The listing builds one solid part. Answer for the finished solid, in the listing's coordinates (mm). A direction names the side the tool comes from. Coordinates: 2 decimals unless noted, no trailing zeros. Order: outer loops, then holes, each group sorted by start corner. A loop starts at its lowest first (then second) coordinate and runs counter-clockwise, first axis right, second up. Notation, with made-up numbers: (1.25, -31) -> (28.25, -31) arc R33 cw to (28.25, 0) -> close; hole circle Ø5 at (27.25, 88). An arc over 180 degrees is marked (long way). Return JSON: item names as keys, results as strings.
from build123d import *

# Parameters (mm, degrees)
F0_W      = 111
F0_H      = 50
F0_W_2    = 99
F0_H_2    = 42
F1_DEPTH  = 1.2
F2_DEPTH  = 41.2
F3_W      = 30.1
F3_H      = 22
F4_DEPTH  = 4
F6_DEPTH  = 20
F7_R      = 1.725
F8_DEPTH  = 114.6
F7_W      = 28
F7_H      = 19.5
F9_DEPTH  = 12
F11_DEPTH = 4
F12_R     = 2


# Not quite as in the source:
# - a feature names something its author has since deleted; it is built from what else it names


with BuildPart() as f1:
    # F0 (on Top) → F1 (new body)
    with BuildSketch(Plane.XY):
        with Locations((55.5, 25)):
            Rectangle(F0_W, F0_H)
        with Locations((55.5, 25)):
            Rectangle(F0_W_2, F0_H_2, mode=Mode.SUBTRACT)
        with Locations((55.5, 25)):
            Rectangle(F0_W_2, F0_H_2)
        with BuildLine():
            ThreePointArc((25.5, 13), (26.9644660941, 16.5355339059), (30.5, 18))
            Line((30.5, 18), (80.5, 18))
            ThreePointArc((80.5, 18), (84.0355339059, 16.5355339059), (85.5, 13))
            Line((85.5, 13), (85.5, 11))
            ThreePointArc((85.5, 11), (84.0355339059, 7.4644660941), (80.5, 6))
            Line((80.5, 6), (30.5, 6))
            ThreePointArc((30.5, 6), (26.9644660941, 7.4644660941), (25.5, 11))
            Line((25.5, 11), (25.5, 13))
        make_face(mode=Mode.SUBTRACT)
    extrude(amount=F1_DEPTH)

    # F0 (on Top) → F2 (join)
    with BuildSketch(Plane.XY):
        with Locations((55.5, 25)):
            Rectangle(F0_W, F0_H)
        with Locations((55.5, 25)):
            Rectangle(F0_W_2, F0_H_2, mode=Mode.SUBTRACT)
    extrude(amount=F2_DEPTH)

    # F3 (on face) → F4 (cut)
    with BuildSketch(Plane(origin=(0, 50, 0), x_dir=(-1, 0, 0), z_dir=(0, 1, 0))):
        with Locations((-55.5, 20.6)):
            Rectangle(F3_W, F3_H)
    extrude(amount=-F4_DEPTH, mode=Mode.SUBTRACT)

    # F5 (on face) → F6 (join)
    with BuildSketch(Plane.XY.offset(41.2)):
        Polygon((0, 50), (0, 23), (6, 23), (6, 46), (105, 46), (105, 23), (111, 23), (111, 50), align=None)
    extrude(amount=F6_DEPTH)

    # F7 (on face) → F8 (cut)
    with BuildSketch(Plane(origin=(0, 0, 0), x_dir=(0, -1, 0), z_dir=(-1, 0, 0))):
        with Locations((-29, 49.2)):
            Circle(F7_R)
        with Locations((-33, 57.2)):
            Circle(F7_R)
    extrude(amount=-F8_DEPTH, mode=Mode.SUBTRACT)

    # F7 (on face) → F9 (cut)
    with BuildSketch(Plane(origin=(0, 0, 0), x_dir=(0, -1, 0), z_dir=(-1, 0, 0))):
        with Locations((-25, 20.6)):
            Rectangle(F7_W, F7_H)
        with Locations((-45, 20.6)):
            Circle(F7_R)
        with Locations((-5, 20.6)):
            Circle(F7_R)
    extrude(amount=-F9_DEPTH, mode=Mode.SUBTRACT)

    # F10 (on face) → F11 (cut)
    with BuildSketch(Plane.YZ.offset(6)):
        Polygon((8.7527767497, 20.6), (6.8763883749, 23.85), (3.1236116251, 23.85), (1.2472232503, 20.6), (3.1236116251, 17.35), (6.8763883749, 17.35), align=None)
        Polygon((43.1236116251, 23.85), (41.2472232503, 20.6), (43.1236116251, 17.35), (46.8763883749, 17.35), (48.7527767497, 20.6), (46.8763883749, 23.85), align=None)
    extrude(amount=F11_DEPTH, mode=Mode.SUBTRACT)

    # F12
    f12_edges = [f1.edges().sort_by_distance(p)[0] for p in [
        (6, 46, 42.525),
        (6, 46, 9.275),
        (105, 46, 31.2),
        (105, 4, 21.2),
        (6, 4, 32.525),
        (6, 4, 9.275),
        (111, 0, 20.6),
        (111, 50, 30.6),
        (0, 50, 30.6),
        (0, 0, 20.6),
    ]]
    fillet(f12_edges, radius=F12_R)


solid = f1.part
1. For faces 5 (the face through (7.5, 46.4, 23.85)), 6 (the face through (70.55, 48, 20)), 7 (the face through (3, 39, 20)), 8 (the face through (51, 2, 41.2)), 9 (the face through (55, 46, 37)), determine the directions among +Z, -Z, +X, -X, +Y, -Y from which every point of the face is accessible in a straight line to the end or side of a thin tool.
Answer block:
{"face 5": "none", "face 6": "+Y", "face 7": "-X", "face 8": "+Z, +X, -X, -Y", "face 9": "+Z"}
2. Each of these flat-tipped pins is pushed along its axis until it touches: pin 1 Ø4 at (x, z) = (62.5, 45) entering from -Y; pin 2 Ø3 at (x, y) = (84.5, 17) entering from +Z; pin 3 Ø3 at (x, z) = (107.5, 50.5) entering from -Y. Where does it stop, or does it pass through?
Answer block:
{"pin 1": "stops at y = 46", "pin 2": "stops at z = 1.2", "pin 3": "stops at y = 23"}
3. The part is cut by section A-A on y = 33. Give the vertices of the cut face in (x, z) (3 decimals).
Answer block:
{"outline": "(0, 0) -> (111, 0) -> (111, 55.475) -> (105, 55.475) -> (105, 1.2) -> (6, 1.2) -> (6, 10.85) -> (0, 10.85) -> close; (0, 30.35) -> (6, 30.35) -> (6, 55.475) -> (0, 55.475) -> close; (0, 58.925) -> (6, 58.925) -> (6, 61.2) -> (0, 61.2) -> close; (105, 58.925) -> (111, 58.925) -> (111, 61.2) -> (105, 61.2) -> close"}
4. Determine the mould class of faces 1 (the face through (26.93, 16.5, 0.59)), 2 (the face through (55, 25, 0)), 3 (the face through (3, 25, 30.35)), 4 (the face through (56, 48, 31.6)) for opening direction Z: pulls with the +Z half, pulls with the -Z half, needs draft (parallel to the pull), parting line crosses it, or undercut.
Answer block:
{"face 1": "needs draft", "face 2": "pulls with the -Z half", "face 3": "undercut", "face 4": "undercut"}
5. The part is cut by section B-B on z = 57.2. Give the vertices of the cut face in (x, y) (3 decimals), and give its area (3 significant figures).
Answer block:
{"outline": "(0, 23) -> (6, 23) -> (6, 31.275) -> (0, 31.275) -> close; (0, 34.725) -> (6, 34.725) -> (6, 44) arc R2 cw to (8, 46) -> (103, 46) arc R2 cw to (105, 44) -> (105, 34.725) -> (111, 34.725) -> (111, 48) arc R2 ccw to (109, 50) -> (2, 50) arc R2 ccw to (0, 48) -> close; (105, 23) -> (111, 23) -> (111, 31.275) -> (105, 31.275) -> close", "area": "679 mm2"}
6. The part is cut by section C-C on x = 17. Give the vertices of the cut face in (y, z).
Answer block:
{"outline": "(0, 0) -> (50, 0) -> (50, 61.2) -> (46, 61.2) -> (46, 1.2) -> (4, 1.2) -> (4, 41.2) -> (0, 41.2) -> close"}
7. Consider line 1 (Z direction, x = 3.2, y = 29) (3 decimals); line 2 (Y direction, x = 1.85, z = 20.6) (3 decimals); line 3 (Z direction, x = 3.85, y = 33) (3 decimals). Determine where each line is inside the solid, lowest interval first. Write a range as from..to.
Answer block:
{"line 1": "z = 0..10.85, 30.35..47.475, 50.925..61.2", "line 2": "y = 0.006..3.275, 6.725..11, 39..43.275, 46.725..49.994", "line 3": "z = 0..10.85, 30.35..55.475, 58.925..61.2"}
8. The part is cut by section D-D on z = 27. Give the vertices of the cut face in (x, y), and give its area (3 significant figures).
Answer block:
{"outline": "(0, 2) arc R2 ccw to (2, 0) -> (109, 0) arc R2 ccw to (111, 2) -> (111, 48) arc R2 ccw to (109, 50) -> (70.55, 50) -> (70.55, 46) -> (103, 46) arc R2 cw to (105, 44) -> (105, 6) arc R2 cw to (103, 4) -> (8, 4) arc R2 cw to (6, 6) -> (6, 11) -> (0, 11) -> close; (0, 39) -> (6, 39) -> (6, 44) arc R2 cw to (8, 46) -> (40.45, 46) -> (40.45, 50) -> (2, 50) arc R2 ccw to (0, 48) -> close", "area": "1,100 mm2"}
